```python
from build123d import *

# Parameters (mm, degrees)
SKETCH1_W           = 15.1
SKETCH1_H           = 9.6
BOSS_EXTRUDE1_DEPTH = 6.9
SKETCH3_R           = 2.25
CUT_EXTRUDE1_DEPTH  = 12.298340586
SKETCH4_R           = 4.15
CUT_EXTRUDE2_DEPTH  = 5.5
SKETCH5_W           = 15.1
SKETCH5_H           = 5
CUT_EXTRUDE3_DEPTH  = 4.1
SKETCH6_W           = 4.5
SKETCH6_H           = 4.1
CUT_EXTRUDE4_DEPTH  = 11.4
SKETCH9_W           = 5
SKETCH9_H           = 2.8
CUT_EXTRUDE5_DEPTH  = 3
FILLET3_R           = 0.5
BOSS_EXTRUDE2_REACH = 14.566
SKETCH10_W          = 2
SKETCH10_H          = 2.6
FILLET4_R           = 4
FILLET5_R           = 0.5
FILLET6_R           = 0.5


with BuildPart() as part:
    # Sketch1 → Boss-Extrude1 (new body)
    with BuildSketch(Plane(origin=(0, 0, 0), x_dir=(1, 0, 0), z_dir=(0, 1, 0))):
        Rectangle(SKETCH1_W, SKETCH1_H)
    extrude(amount=BOSS_EXTRUDE1_DEPTH)

    # Sketch3 → Cut-Extrude1 (cut, through all)
    with BuildSketch(Plane(origin=(0, 6.9, 0), x_dir=(1, 0, 0), z_dir=(0, 1, 0))):
        with Locations(Location((0, 0, 0), (0, 0, 270))):
            Circle(SKETCH3_R)
    extrude(amount=-CUT_EXTRUDE1_DEPTH, mode=Mode.SUBTRACT)

    # Sketch4 → Cut-Extrude2 (cut)
    with BuildSketch(Plane(origin=(0, 6.9, 0), x_dir=(1, 0, 0), z_dir=(0, 1, 0))):
        with Locations(Location((0, 0, 0), (0, 0, 270))):
            Circle(SKETCH4_R)
    extrude(amount=-CUT_EXTRUDE2_DEPTH, mode=Mode.SUBTRACT)

    # Sketch5 → Cut-Extrude3 (cut)
    with BuildSketch(Plane(origin=(0, 6.9, 0), x_dir=(1, 0, 0), z_dir=(0, 1, 0))):
        Rectangle(SKETCH5_W, SKETCH5_H)
    extrude(amount=-CUT_EXTRUDE3_DEPTH, mode=Mode.SUBTRACT)

    # Sketch6 → Cut-Extrude4 (cut, symmetric)
    with BuildSketch(Plane.XY):
        with Locations((0, 4.85)):
            Rectangle(SKETCH6_W, SKETCH6_H)
    extrude(amount=CUT_EXTRUDE4_DEPTH, both=True, mode=Mode.SUBTRACT)

    # Sketch9 → Cut-Extrude5 (cut)
    with BuildSketch(Plane.ZY.offset(7.55)):
        with Locations((0, 1.4)):
            Rectangle(SKETCH9_W, SKETCH9_H)
    cut_extrude5 = extrude(amount=-CUT_EXTRUDE5_DEPTH, mode=Mode.SUBTRACT)

    # Fillet3
    fillet3_edges = [part.edges().sort_by_distance(p)[0] for p in [
        (7.55, 3.45, 4.8),
        (-7.55, 3.45, 4.8),
        (-7.55, 3.45, -4.8),
        (7.55, 3.45, -4.8),
    ]]
    fillet(fillet3_edges, radius=FILLET3_R)

    # Sketch10 → Boss-Extrude2 (add, up to next)
    with BuildSketch(Plane.XY.offset(-2.5), mode=Mode.PRIVATE) as boss_extrude2_sk1:
        with Locations((-6.55, 5.6)):
            Rectangle(SKETCH10_W, SKETCH10_H)
    boss_extrude2_tool1 = extrude(boss_extrude2_sk1.sketch, amount=BOSS_EXTRUDE2_REACH, mode=Mode.PRIVATE) - part.part
    boss_extrude2 = boss_extrude2_tool1.solids().sort_by_distance((-6.55, 5.6, -2.5))[0]
    add(boss_extrude2)

    # Mirror1: Cut-Extrude5, Boss-Extrude2 across plane
    add(cut_extrude5.mirror(Plane(origin=(0, 0, 0), x_dir=(0, 0, 1), z_dir=(1, 0, 0))), mode=Mode.SUBTRACT)
    add(boss_extrude2.mirror(Plane(origin=(0, 0, 0), x_dir=(0, 0, 1), z_dir=(1, 0, 0))))

    # Fillet4
    # the kernel refuses this fillet: 4 mm, written as the material it takes off along each edge
    with BuildSketch(Plane(origin=(2.25, 6.9, -14.8), x_dir=(0, -1, 0), z_dir=(0, 0, 1)), Plane(origin=(-2.25, 6.9, 6.512880845), x_dir=(0, -1, 0), z_dir=(0, 0, -1))) as fillet4_piece_1:
        with BuildLine():
            CenterArc((FILLET4_R, FILLET4_R), FILLET4_R, 180, 90)
            Line((0, FILLET4_R), (0, 0))
            Line((0, 0), (FILLET4_R, 0))
        make_face()
    extrude(amount=21.312880845, mode=Mode.SUBTRACT)

    # Fillet5
    fillet5_edges = [part.edges().sort_by_distance(p)[0] for p in [
        (6.65, 6.9, -4.8),
        (7.403553391, 6.9, -4.653553391),
        (-6.65, 6.9, 4.8),
        (7.403553391, 6.9, 4.653553391),
        (-7.403553391, 6.9, 4.653553391),
        (-7.403553391, 6.9, -4.653553391),
        (6.65, 6.9, 4.8),
        (2.25, 2.85, 4.8),
        (3.421572875, 5.728427125, 4.8),
        (-3.421572875, 5.728427125, 4.8),
        (-6.65, 6.9, -4.8),
        (-2.25, 2.85, -4.8),
        (-3.421572875, 5.728427125, -4.8),
        (3.421572875, 5.728427125, -4.8),
        (7.55, 6.9, 0),
        (-7.55, 6.9, 0),
        (-2.25, 2.85, 4.8),
        (2.25, 2.85, -4.8),
    ]]
    fillet(fillet5_edges, radius=FILLET5_R)

    # Fillet6
    fillet6_edges = [part.edges().sort_by_distance(p)[0] for p in [
        (-7.55, 4.3, 0),
        (7.55, 4.3, 0),
    ]]
    fillet(fillet6_edges, radius=FILLET6_R)


solid = part.part
```
Could you check a few things on this model? Use its own coordinates, in mm. A direction names the side the tool comes from. Round coordinates to 2 decimals unless told otherwise and drop trailing zeros. Loops run counter-clockwise (first coordinate to the right, second up) from the corner with the lowest first, then second, coordinate; pieces in that order, holes last. Notation, with made-up numbers: (24.25, 44) -> (38.25, 44) arc R22 ccw to (38.25, 57) -> close; hole circle Ø3 at (-23.75, -28.5). An arc over 180 degrees is marked (long way). Put each result on its own line as item: value.
Q1. I want a section at C-C on y = 2.5. Write out the boundary of the cut face in (x, z).
Checks:
outline: (-7.55, -4.3) arc R0.5 ccw to (-7.05, -4.8) -> (7.05, -4.8) arc R0.5 ccw to (7.55, -4.3) -> (7.55, -2.5) -> (4.55, -2.5) -> (4.55, 2.5) -> (7.55, 2.5) -> (7.55, 4.3) arc R0.5 ccw to (7.05, 4.8) -> (-7.05, 4.8) arc R0.5 ccw to (-7.55, 4.3) -> (-7.55, 2.5) -> (-4.55, 2.5) -> (-4.55, -2.5) -> (-7.55, -2.5) -> close; hole circle Ø8.3 at (0, 0)
Q2. I want a section at D-D on x = 1.75. Write out the boundary of the cut face in (y, z).
Checks:
outline: (0, -4.8) -> (2.8, -4.8) -> (2.8, -3.76) -> (1.4, -3.76) -> (1.4, -1.41) -> (0, -1.41) -> close; (0, 1.41) -> (1.4, 1.41) -> (1.4, 3.76) -> (2.8, 3.76) -> (2.8, 4.8) -> (0, 4.8) -> close
Q3. For pin 1 Ø0.6 at (x, z) = (-4, 1) entering from +Y; pin 2 Ø1.6 at (x, z) = (-6, 0.5) entering from -Y, each with a flat end and sliding along its axis, tell me the tip position at first contact or that it passes through.
Checks:
pin 1: y = 2.8
pin 2: y = 4.3
Q4. I want a section at B-B on x = 0. Write out the boundary of the cut face in (y, z).
Checks:
outline: (0, -4.8) -> (2.8, -4.8) -> (2.8, -4.15) -> (1.4, -4.15) -> (1.4, -2.25) -> (0, -2.25) -> close; (0, 2.25) -> (1.4, 2.25) -> (1.4, 4.15) -> (2.8, 4.15) -> (2.8, 4.8) -> (0, 4.8) -> close
Q5. I want a section at A-A on z = 0. Write out the boundary of the cut face in (x, y).
Checks:
outline: (-7.55, 4.8) arc R0.5 ccw to (-7.05, 4.3) -> (-5.55, 4.3) -> (-5.55, 6.84) arc R4 ccw to (-6.25, 6.9) -> (-7.05, 6.9) arc R0.5 ccw to (-7.55, 6.4) -> close; (-4.55, 0) -> (-2.25, 0) -> (-2.25, 1.4) -> (-4.15, 1.4) -> (-4.15, 2.8) -> (-4.55, 2.8) -> close; (2.25, 0) -> (4.55, 0) -> (4.55, 2.8) -> (4.15, 2.8) -> (4.15, 1.4) -> (2.25, 1.4) -> close; (5.55, 4.3) -> (7.05, 4.3) arc R0.5 ccw to (7.55, 4.8) -> (7.55, 6.4) arc R0.5 ccw to (7.05, 6.9) -> (6.25, 6.9) arc R4 ccw to (5.55, 6.84) -> close
Q6. Please list where these lines run through material, in increasing order: line 1 (Z direction, x = 3.75, y = 5); line 2 (X direction, y = 0.7, z = 0); line 3 (Z direction, x = -2.5, y = 1.5). Write a range as from..to.
Checks:
line 1: -4.8..-2.5, 2.5..4.8
line 2: -4.55..-2.25, 2.25..4.55
line 3: -4.8..-3.31, 3.31..4.8
Q7. Which directions (+Z, -Z, +X, -X, +Y, -Y) give clear straight access to the entire face, cutting with the end or side of a thin tool? Please do faces 5 (the flat face through (4.55, 1, 0)), 6 (the flat face through (4.34, 2.8, -0.04)), 7 (the flat face through (5, 3, -2.5)), 8 (the cylindrical face through (-5.95, 6.89, 0.06)), 9 (the flat face through (-5.55, 6, 0)).
Checks:
face 5: +X, +Y, -Y
face 6: +X, -X, +Y
face 7: none
face 8: +Z, -Z, +Y
face 9: +Y, -Y
Q8. Thinking about a two-plate mould opening in Z: for faces 1 (the flat face through (5, 3, 2.5)), 2 (the flat face through (0, 2, -4.8)), 3 (the flat face through (7.55, 5, 0)), 4 (the flat face through (-4.55, 1, 0)), which applies, pulls with the +Z half, pulls with the -Z half, needs draft (parallel to the pull), parting line crosses it, or undercut?
Checks:
face 1: undercut
face 2: pulls with the -Z half
face 3: needs draft
face 4: undercut
